from build123d import *

# Parameters (mm, degrees)
SZKIC1_W = 11
SZKIC1_H = 66
SZKIC2_W = 11
SZKIC2_H = 66


with BuildPart() as part:
    # Szkic1 → Obrót1 (revolve)
    with BuildSketch(Plane.XY):
        with Locations((-5.5, 0)):
            Rectangle(SZKIC1_W, SZKIC1_H)
    revolve(axis=Axis((0, 33, 0), (0, -1, 0)))

    # Szkic2 → Obrót2 (revolve)
    with BuildSketch(Plane(origin=(0, 0, 0), x_dir=(1, 0, 0), z_dir=(0, 1, 0))):
        with Locations((-5.5, 0)):
            Rectangle(SZKIC2_W, SZKIC2_H)
    revolve(axis=Axis((0, 0, -33), (0, 0, 1)))


solid = part.part
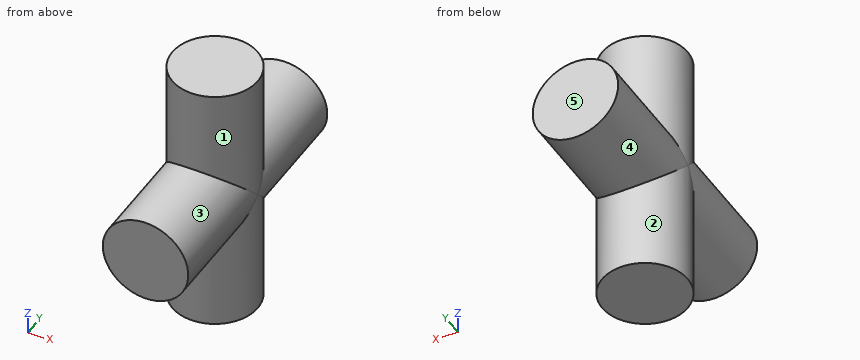
Can you work these out from the model? Positions are in its coordinate system, mm. Face numbers are marked on the shaded views. A direction names the side the tool comes from. Give positions to 0.01 mm unless a question says otherwise; leave off trailing zeros. Order: outer loops, then holes, each group sorted by start corner. A loop starts at its lowest first (then second) coordinate and runs counter-clockwise, first axis right, second up. Notation, with made-up numbers: (28.25, 32.5) - (66.25, 32.5) arc R24 ccw to (66.25, 42.5) - close; hole circle Ø4 at (20, -27.5). An arc over 180 degrees is marked (long way). Write each question's results on one line, items separated by ' | '.
1) Please list where these lines run through material, in increasing order: line 1 along Z through (x, y) = (-0.5, -12); line 2 along Y through (x, z) = (-1.25, -23); line 3 along Y through (x, z) = (-4.25, 15.5). Write a range as [from, to].
Final values:
line 1: z = [-10.99, 10.99] | line 2: y = [-10.93, 10.93] | line 3: y = [-10.15, 10.15]
2) Suppose I cut it at A-A, the plane x = 0. Write out the boundary of the cut face in (y, z).
Final values:
outline: (-33, -11) - (-11, -11) - (-11, -33) - (11, -33) - (11, -11) - (33, -11) - (33, 11) - (11, 11) - (11, 33) - (-11, 33) - (-11, 11) - (-33, 11) - close
3) On a 3-axis mill with a long thin cutter (end or side, diameter ignored), from which of +Z, -Z, +X, -X, +Y, -Y can I reach the whole of each face in a straight line? I mean the marked faces 1, 2, 3, 4 and 5. Say none if no direction works.
Final values:
face 1: +Z | face 2: -Z | face 3: -Y | face 4: +Y | face 5: +Z, -Z, +X, -X, +Y
4) I'm going to push flat-ended pins straight in: pin 1 Ø4 at (x, y) = (0, 15) entering from +Z; pin 2 Ø3 at (x, z) = (2, -23.5) entering from +Y; pin 3 Ø10 at (x, z) = (-4, -24) entering from -Y. Where does each tip first touch, or does it pass through?
Final values:
pin 1: stops at z = 11 | pin 2: stops at y = 10.99 | pin 3: stops at y = -11
5) Suppose I cut it at D-D, the plane x = 8. Write out the boundary of the cut face in (y, z).
Final values:
outline: (-33, -7.55) - (-7.55, -7.55) - (-7.55, -33) - (7.55, -33) - (7.55, -7.55) - (33, -7.55) - (33, 7.55) - (7.55, 7.55) - (7.55, 33) - (-7.55, 33) - (-7.55, 7.55) - (-33, 7.55) - close
6) Suppose I cut it at C-C, the plane z = -9.5. Write out the boundary of the cut face in (x, y), then the cut area to 3 significant figures.
Final values:
outline: (-5.55, -33) - (5.55, -33) - (5.55, -9.5) arc R11 ccw to (5.55, 9.5) - (5.55, 33) - (-5.55, 33) - (-5.55, 9.5) arc R11 ccw to (-5.55, -9.5) - close | area: 879 mm^2
7) Suppose I cut it at B-B, the plane y = 7.5. Write out the boundary of the cut face in (x, z), then the cut area to 3 significant figures.
Final values:
outline: (-8.05, -33) - (8.05, -33) - (8.05, -7.5) arc R11 ccw to (8.05, 7.5) - (8.05, 33) - (-8.05, 33) - (-8.05, 7.5) arc R11 ccw to (-8.05, -7.5) - close | area: 1,120 mm^2
